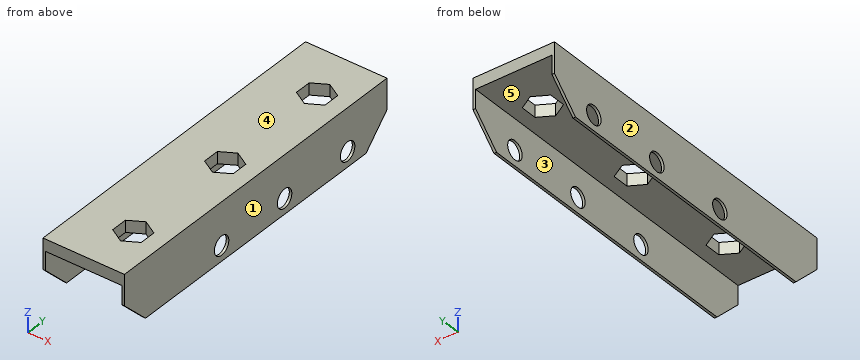
from build123d import *

# Parameters (mm, degrees)
BOSS_EXTRUDE1_DEPTH     = 100
CUT_EXTRUDE1_DEPTH      = 105.235310716
CUT_EXTRUDE1_DEPTH_BACK = 105.235310716
M5_CLEARANCE_HOLE1_D    = 5.5
CHAMFER1_SIZE           = 8


with BuildPart() as part:
    # Sketch1 → Boss-Extrude1 (new body)
    with BuildSketch(Plane(origin=(0, 0, 0), x_dir=(1, 0, 0), z_dir=(0, 1, 0))):
        Polygon((0, 0), (0, 17), (0.75, 17), (0.75, 3.5), (23.25, 3.5), (23.25, 17), (24, 17), (24, 0), align=None)
    extrude(amount=BOSS_EXTRUDE1_DEPTH)

    # Sketch2 → Cut-Extrude1 (cut, two sides: drawn at the far end of the back side and taken through both)
    with BuildSketch(Plane.XY.offset(-CUT_EXTRUDE1_DEPTH_BACK)):
        Polygon((10.8, 52.424871131), (10.8, 47.575128869), (15, 45.150257739), (19.2, 47.575128869), (19.2, 52.424871131), (15, 54.849742261), align=None)
        Polygon((19.2, 12.575128869), (19.2, 17.424871131), (15, 19.849742261), (10.8, 17.424871131), (10.8, 12.575128869), (15, 10.150257739), align=None)
        Polygon((10.8, 87.424871131), (10.8, 82.575128869), (15, 80.150257739), (19.2, 82.575128869), (19.2, 87.424871131), (15, 89.849742261), align=None)
    extrude(amount=CUT_EXTRUDE1_DEPTH + CUT_EXTRUDE1_DEPTH_BACK, mode=Mode.SUBTRACT)

    # M5 Clearance Hole1 (through all)
    with Locations(Plane(origin=(24, 0, 0), x_dir=(0, 0, -1), z_dir=(1, 0, 0))):
        with Locations((12.5, 85), (12.5, 37), (12.5, 61)):
            Hole(M5_CLEARANCE_HOLE1_D / 2)

    # Chamfer1
    chamfer1_edges = [part.edges().sort_by_distance(p)[0] for p in [
        (23.625, 0, -17),
        (23.625, 100, -17),
        (0.375, 100, -17),
        (0.375, 0, -17),
    ]]
    chamfer(chamfer1_edges, length=CHAMFER1_SIZE)


solid = part.part
Design review of the part built by this model. Coordinates are the model's own, in mm. Face numbers are marked on the shaded views. A direction names the side the tool comes from. Round coordinates to 2 decimals unless told otherwise and drop trailing zeros. Write each loop counter-clockwise with the first axis right and the second up, starting at its lowest first coordinate (ties: lowest second). Pieces come first, ordered by that corner, then holes. Notation, with made-up numbers: (-26, 26.5) -> (-3, 26.5) arc R9 cw to (-3, 32.5) -> close; hole circle Ø3 at (-34.5, 48). An arc over 180 degrees is marked (long way). One line per question, with ' | ' between items.
(1) Draft analysis for pull direction X (two halves, no side actions). For the marked faces 1, 2 and 3, state which applies: released by +X, released by -X, zero draft, split by the parting line, or undercut.
Result sheet:
face 1: released by +X | face 2: released by -X | face 3: undercut
(2) Take a section at B-B, the plane z = -5.5. State the section outline as (x, y) points, and give its area (3 significant figures).
Result sheet:
outline: (0, 0) -> (0.75, 0) -> (0.75, 100) -> (0, 100) -> close; (23.25, 0) -> (24, 0) -> (24, 100) -> (23.25, 100) -> close | area: 150 mm2
(3) Take a section at D-D, the plane z = -12.5. State how many separate pieces and enclosed holes the cut face has, and give its area (3 significant figures).
Result sheet:
separate pieces: 8 | enclosed holes: 0 | area: 115 mm2
(4) Wall thickness on line 1 (X direction, y = 70, z = -12.5); line 2 (Y direction, x = 23.45, z = -12.5); line 3 (X direction, y = 48, z = -1): over which ranges is each line inside the solid? List them lowest first. Write a range as [from, to].
Result sheet:
line 1: [0, 0.75], [23.25, 24] | line 2: [3.5, 34.25], [39.75, 58.25], [63.75, 82.25], [87.75, 96.5] | line 3: [0, 10.8], [19.2, 24]
(5) Take a section at A-A, the plane y = 85. State the section outline as (x, z) points.
Result sheet:
outline: (0, -17) -> (0.75, -17) -> (0.75, -15.25) -> (0, -15.25) -> close; (0, -9.75) -> (0.75, -9.75) -> (0.75, -3.5) -> (10.8, -3.5) -> (10.8, 0) -> (0, 0) -> close; (19.2, -3.5) -> (23.25, -3.5) -> (23.25, -9.75) -> (24, -9.75) -> (24, 0) -> (19.2, 0) -> close; (23.25, -17) -> (24, -17) -> (24, -15.25) -> (23.25, -15.25) -> close
(6) Machinability: for the marked faces 4 and 5, which of the approach directions +Z, -Z, +X, -X, +Y, -Y give a long, thin tool a straight path to every point of the face, cutting with its end or side? Answer none if there is none.
Result sheet:
face 4: +Z, +X, -X, +Y, -Y | face 5: -Z, +Y, -Y
(7) Insertion check: P1, Ø11, axis at x = 8, y = 71.5, coming from the -Z side; P2, Ø5, axis at y = 61, z = -12.5, coming from the +X side. Each pin has a flat end and moves straight along its axis. Give the tip position at first contact, or say it passes through.
Result sheet:
P1: z = -3.5 | P2: through
(8) Take a section at C-C, the plane y = 61. State the section outline as (x, z) points, and give its area (3 significant figures).
Result sheet:
outline: (0, -17) -> (0.75, -17) -> (0.75, -15.25) -> (0, -15.25) -> close; (0, -9.75) -> (0.75, -9.75) -> (0.75, -3.5) -> (23.25, -3.5) -> (23.25, -9.75) -> (24, -9.75) -> (24, 0) -> (0, 0) -> close; (23.25, -17) -> (24, -17) -> (24, -15.25) -> (23.25, -15.25) -> close | area: 96.0 mm2
